The model under review builds one solid part; all positions refer to its coordinate system, in mm. A direction names the side the tool comes from. Coordinates: 2 decimals unless noted, no trailing zeros. Write each loop counter-clockwise with the first axis right and the second up, starting at its lowest first coordinate (ties: lowest second). Pieces come first, ordered by that corner, then holes.
Autodesk Inventor part; units mm, degrees
ref_plane "YZ Plane" through (0, 0, 0) normal (1, 0, 0) x (0, 1, 0)
ref_plane "XZ Plane" through (0, 0, 0) normal (0, 1, 0) x (-1, 0, 0)
ref_plane "XY Plane" through (0, 0, 0) normal (0, 0, 1) x (1, 0, 0)
sketch "Sketch1" plane through (0, 0, 0) normal (1, 0, 0) x (0, 1, 0)
  circle A0 centre (0, 0) radius 7
  line L0 (0, -11) -> (-31, -11)
  line L1 (-31, -11) -> (-31, 24)
  line L2 (-11, -11) -> (-11, 24)
  line L3 (-31, 24) -> (-11, 24)
  line L4 (0, -20.9958) -> (0, 31.4993)
  arc A1 (0, -11) -> (7.1808, 8.3329) centre (0, 0) ccw
  line L5 (-11, 24) -> (7.1808, 8.3329)
  dimension "d0" = 14
  dimension "d3" = 11
  dimension "d4" = 35
  dimension "d6" = 22
  dimension "d7" = 31
extrude "Extrusion1" add sketch "Sketch1" along normal blind 9.5813 contours A0 L4 L5 A1 | A0 L4 L0 L2 L5
extrude "Extrusion2" add sketch "Sketch1" along normal blind 4.5813 contours A0 L4 | L4 A0
extrude "Extrusion3" add sketch "Sketch1" against normal blind 6
sketch "Sketch2" plane through (-6, 0, 0) normal (-1, 0, 0) x (0, 0, 1)
  circle A0 centre (6.5, -21) radius 2
  line L0 (-11, -31) -> (24, -31)
  line L1 (-11, 0) -> (-11, -31)
  point P0 (0, 0)
  dimension "d14" = 4
  dimension "d15" = 10
  dimension "d16" = 17.5
extrude "Extrusion4" cut sketch "Sketch2" against normal blind 10
chamfer "Chamfer1" distance 3 angle 45 1 edges at (-6, -21, 4.5)
properties part number "bearing_holder_v2_left"
Item 1: Take a section at D-D, the plane y = 6. Write out the cut boundary in (x, z).
Solved:
outline: (-6, -9.22) - (9.58, -9.22) - (9.58, -3.61) - (4.58, -3.61) - (4.58, 3.61) - (9.58, 3.61) - (9.58, 9.35) - (-6, 9.35) - close
Item 2: For pin 1 (6 mm diameter, centred on y = -20, z = 9, fed in from +X); pin 2 (7.5 mm diameter, centred on x = 4.5, z = 15, fed in from -Y); pin 3 (6 mm diameter, centred on y = 3, z = -2, fed in from +X), all flat-tipped, find the tip position at first contact; note any pin that passes through.
Solved:
pin 1: stops at x = 0
pin 2: stops at y = -11
pin 3: stops at x = 4.58
Item 3: Take a section at B-B, the plane y = -5. Write out the cut boundary in (x, z), plus the area to 3 significant figures.
Solved:
outline: (-6, -11) - (9.58, -11) - (9.58, -4.9) - (4.58, -4.9) - (4.58, 4.9) - (9.58, 4.9) - (9.58, 18.83) - (-6, 18.83) - close
area: 416 mm2
Item 4: Take a section at C-C, the plane z = 0. Write out the cut boundary in (x, y).
Solved:
outline: (-6, -31) - (0, -31) - (0, -11) - (9.58, -11) - (9.58, -7) - (4.58, -7) - (4.58, 7) - (9.58, 7) - (9.58, 11) - (-6, 11) - close
Item 5: To check wall thickness, follow line 1 along Y through (x, z) = (5.95, 0); line 2 along X through (y, z) = (-13, 20); line 3 along Y through (x, z) = (-2, 8). State the ranges of each line that lie inside material, in increasing order.
Solved:
line 1: y = -11 to -7, 7 to 11
line 2: x = -6 to 0
line 3: y = -31 to -22.32, -19.68 to 7.55
Item 6: Machinability: for faces 1 (the face through (9.581, -3, 7)), 2 (the face through (0, -23.4, 6.7)), 3 (the face through (4.581, 0, 0)), which of the approach directions +Z, -Z, +X, -X, +Y, -Y give a long, thin tool a straight path to every point of the face, cutting with its end or side? Answer none if there is none.
Solved:
face 1: +Z, -Z, +X, +Y, -Y
face 2: +Z, -Z, +X, -Y
face 3: +X
Item 7: Take a section at A-A, the plane z = 6.5. Write out the cut boundary in (x, y).
Solved:
outline: (-6, -31) - (0, -31) - (0, -23) - (-3, -23) - (-6, -26) - close; (-6, -16) - (-3, -19) - (0, -19) - (0, -11) - (9.58, -11) - (9.58, -2.6) - (4.58, -2.6) - (4.58, 2.6) - (9.58, 2.6) - (9.58, 8.87) - (-6, 8.87) - close
